Source: CAD feature listing. Evaluate the final solid. Frame: model axes, mm. A direction names the side the tool comes from. Round coordinates to 2 decimals unless told otherwise and drop trailing zeros. Loops run counter-clockwise (first coordinate to the right, second up) from the corner with the lowest first, then second, coordinate; pieces in that order, holes last. Notation, with made-up numbers: M 84,37 L 108,37 A19 cw 108,50 Z; hole C 20,8.5 d10. An arc over 180 degrees is marked long. One line per item, written item: value.
from build123d import *

# Parameters (mm, degrees)
SKETCH1_R           = 1.70053
BOSS_EXTRUDE1_DEPTH = 6.35


with BuildPart() as part:
    # Sketch1 → Boss-Extrude1 (new body)
    with BuildSketch(Plane(origin=(0, 0, 0), x_dir=(1, 0, 0), z_dir=(0, 1, 0))):
        with BuildLine():
            Line((100.72984212, 33.562647915), (94.097535909, 42.20603765))
            ThreePointArc((94.097535909, 42.20603765), (84.176111379, 47.17383179), (74.137013371, 42.448352501))
            ThreePointArc((74.137013371, 42.448352501), (0, 7.00024), (-74.137013371, 42.448352501))
            ThreePointArc((-74.137013371, 42.448352501), (-84.176111379, 47.17383179), (-94.097535909, 42.20603765))
            Line((-94.097535909, 42.20603765), (-100.72984212, 33.562647915))
            ThreePointArc((-100.72984212, 33.562647915), (-96.085326852, 27.20294582), (-91.039926176, 21.156354646))
            Line((-91.039926176, 21.156354646), (-81.532472576, 33.546709409))
            Line((-81.532472576, 33.546709409), (-63.396415217, 19.630423142))
            Line((-63.396415217, 19.630423142), (-45.260357858, 5.714136875))
            Line((-45.260357858, 5.714136875), (-54.767811458, -6.676217888))
            ThreePointArc((-54.767811458, -6.676217888), (-51.042995201, -8.470575753), (-47.259480127, -10.137606043))
            Line((-47.259480127, -10.137606043), (-45.332616871, -1.072427153))
            Line((-45.332616871, -1.072427153), (-0.611708566, -10.578149657))
            Line((-0.611708566, -10.578149657), (0.611708566, -10.578149657))
            Line((0.611708566, -10.578149657), (45.332616871, -1.072427153))
            Line((45.332616871, -1.072427153), (47.259480127, -10.137606043))
            ThreePointArc((47.259480127, -10.137606043), (51.042995201, -8.470575753), (54.767811458, -6.676217888))
            Line((54.767811458, -6.676217888), (45.260357858, 5.714136875))
            Line((45.260357858, 5.714136875), (63.396415217, 19.630423142))
            Line((63.396415217, 19.630423142), (81.532472576, 33.546709409))
            Line((81.532472576, 33.546709409), (91.039926176, 21.156354646))
            ThreePointArc((91.039926176, 21.156354646), (96.085326852, 27.20294582), (100.72984212, 33.562647915))
        make_face()
        with Locations(Location((83.82, 40.64, 0), (0, 0, 270))):
            Circle(SKETCH1_R, mode=Mode.SUBTRACT)
        with Locations(Location((-83.82, 40.64, 0), (0, 0, 90))):
            Circle(SKETCH1_R, mode=Mode.SUBTRACT)
        with Locations(Location((0, 0, 0), (0, 0, 270))):
            Circle(SKETCH1_R, mode=Mode.SUBTRACT)
    extrude(amount=BOSS_EXTRUDE1_DEPTH)


solid = part.part
1. Section query B-B (y = 3.5). Return the cut outline in (x, z).
Report:
outline: M -100.73,-33.56 L -94.1,-42.21 A12.7 ccw -74.14,-42.45 A95.25 cw 74.14,-42.45 A12.7 ccw 94.1,-42.21 L 100.73,-33.56 A121.92 ccw 91.04,-21.16 L 81.53,-33.55 L 45.26,-5.71 L 54.77,6.68 A121.92 ccw 47.26,10.14 L 45.33,1.07 L 0.61,10.58 L -0.61,10.58 L -45.33,1.07 L -47.26,10.14 A121.92 ccw -54.77,6.68 L -45.26,-5.71 L -81.53,-33.55 L -91.04,-21.16 A121.92 ccw Z; hole C -83.82,-40.64 d3.4; hole C 0,0 d3.4; hole C 83.82,-40.64 d3.4
2. Pin query (flat end, axial travel): pin 1 (1.5 mm diameter, centred on x = 17.5, y = 1, fed in from -Z); pin 2 (2 mm diameter, centred on x = -75, y = 0.5, fed in from +Z); pin 3 (2 mm diameter, centred on y = 4, z = -5.5, fed in from +X). Return the tip coordinate at first contact, or that it passes through.
Report:
pin 1: stops at z = -8.76
pin 2: stops at z = -27.77
pin 3: stops at x = 46.28
3. Section query D-D (x = -42.5). Return the cut outline in (y, z), and give its area (3 significant figures).
Report:
outline: M 0,-17.01 L 6.35,-17.01 L 6.35,1.67 L 0,1.67 Z
area: 119 mm2
4. Pull-direction query (X, two-part tool) for faces 1 (the face through (-84.015, 3.131, -47.175)), 2 (the face through (-85.506, 3.131, -40.419)), 3 (the face through (96.02, 3.13, -27.12)), 4 (the face through (-97.4, 3.1, -37.9)); classes: released by +X, released by -X, zero draft, split by the parting line, or undercut.
Report:
face 1: undercut
face 2: undercut
face 3: released by +X
face 4: released by -X
5. Section query C-C (x = 83.82). Return the cut outline in (y, z), and give its area (3 significant figures).
Report:
outline: M 0,-47.17 L 6.35,-47.17 L 6.35,-42.34 L 0,-42.34 Z; M 0,-38.94 L 6.35,-38.94 L 6.35,-30.57 L 0,-30.57 Z
area: 83.9 mm2
6. Ray query, line 1 (X direction, y = 3.5, z = -40.64); line 2 (X direction, y = 1.5, z = -41); line 3 (Z direction, x = -83.82, y = 2.75). Return the intervals inside material, ascending. Write a range as [from, to].
Report:
line 1: x = [-95.3, -85.52], [-82.12, -72.64], [72.64, 82.12], [85.52, 95.3]
line 2: x = [-95.02, -85.48], [-82.16, -72.94], [72.94, 82.16], [85.48, 95.02]
line 3: z = [-47.17, -42.34], [-38.94, -30.57]
7. Section query A-A (z = -27). Return the cut outline in (x, y), and give its area (3 significant figures).
Report:
outline: M -95.93,0 L -86.56,0 L -86.56,6.35 L -95.93,6.35 Z; M -73,0 L -58.39,0 L -58.39,6.35 L -73,6.35 Z; M 58.39,0 L 73,0 L 73,6.35 L 58.39,6.35 Z; M 86.56,0 L 95.93,0 L 95.93,6.35 L 86.56,6.35 Z
area: 304 mm2
8. Reachability of faces 5 (the face through (50.99, 3.131, 8.495)), 6 (the face through (-86.353, 3.131, -27.265)), 7 (the face through (63.143, 3.131, -19.436)) from +Z, -Z, +X, -X, +Y, -Y: full face, straight path, thin tool, end or side. Return the list, or none.
Report:
face 5: +Z, +X, +Y, -Y
face 6: +Z, +Y, -Y
face 7: +Y, -Y
